```python
from build123d import *

# Parameters (mm, degrees)
REVOLVE1_ANGLE          = 180
SKETCH2_R               = 2.25
CUT_EXTRUDE1_DEPTH      = 15
CUT_EXTRUDE2_DEPTH      = 5
CUT_EXTRUDE2_DEPTH_BACK = 32.176914536
SKETCH4_W               = 3
SKETCH4_H               = 7


with BuildPart() as part:
    # Sketch1 → Revolve1 (revolve)
    with BuildSketch(Plane(origin=(0, 0, 0), x_dir=(0, 0, -1), z_dir=(1, 0, 0))):
        with BuildLine():
            Line((-18, 0), (18, 0))
            ThreePointArc((18, 0), (0, -18), (-18, 0))
        make_face()
    revolve(axis=Axis((0, 0, 18), (0, 0, -1)), revolution_arc=REVOLVE1_ANGLE)

    # Sketch2 → Cut-Extrude1 (cut)
    with BuildSketch(Plane(origin=(0, 0, 0), x_dir=(0, 0, -1), z_dir=(1, 0, 0))):
        with Locations(Location((0, 0, 0), (0, 0, 90))):
            Circle(SKETCH2_R)
    extrude(amount=-CUT_EXTRUDE1_DEPTH, mode=Mode.SUBTRACT)

    # Sketch4 → Cut-Extrude2 (cut, two sides: drawn at the far end of the back side and taken through both)
    with BuildSketch(Plane(origin=(0, 0, 0), x_dir=(1, 0, 0), z_dir=(0, 1, 0)).offset(-CUT_EXTRUDE2_DEPTH_BACK)):
        with Locations((-7.141823204, 0)):
            Rectangle(SKETCH4_W, SKETCH4_H)
    extrude(amount=CUT_EXTRUDE2_DEPTH + CUT_EXTRUDE2_DEPTH_BACK, mode=Mode.SUBTRACT)


solid = part.part
```
Read the model definition and answer for the solid it produces. Units are mm, in the model's axes. A direction names the side the tool comes from. Round coordinates to 2 decimals unless told otherwise and drop trailing zeros. Write each loop counter-clockwise with the first axis right and the second up, starting at its lowest first coordinate (ties: lowest second). Pieces come first, ordered by that corner, then holes. Notation, with made-up numbers: (-16.5, 27) - (6.5, 27) arc R27 ccw to (6.5, 57) - close; hole circle Ø11 at (78, 86.25). An arc over 180 degrees is marked (long way). Use CSV: the item, a comma, the result in double quotes.
Q1. Find section C-C, the plane y = -13.5. Write down the section's boundary in (x, z), then the cut area to 3 significant figures.
Values:
outline,"(0, -11.91) - (0, 11.91) arc R11.91 ccw to start; hole (-8.64, -3.5) - (-5.64, -3.5) - (-5.64, 3.5) - (-8.64, 3.5) - close"
area,"202 mm²"
Q2. Straight lines are drawn through the part: line 1 along Z through (x, y) = (-7, -15); line 2 along Z through (x, y) = (-11.75, 0); line 3 along X through (y, z) = (-8, 0.5). For each, find the intervals that lie inside material, in ascending order.
Values:
line 1,"z = -7.07 to -3.5, 3.5 to 7.07"
line 2,"z = -13.64 to -2.25, 2.25 to 13.64"
line 3,"x = -16.12 to -8.64, -5.64 to 0"
Q3. Each of these flat-tipped pins is pushed along its axis until it touches: pin 1 Ø1.5 at (x, z) = (-14, 0.5) entering from -Y; pin 2 Ø2.5 at (y, z) = (0, 0) entering from +X; pin 3 Ø2 at (y, z) = (-6.5, -0.5) entering from -X; pin 4 Ø1.5 at (x, z) = (-15.5, 13.5) entering from -Y. Where does it stop, or does it pass through?
Values:
pin 1,"stops at y = -12.17"
pin 2,"stops at x = -15"
pin 3,"stops at x = -17.13"
pin 4,"passes through"
Q4. Determine the mould class of faces 3 (the cylindrical face through (-2.781, 2.146, 0.676)), 4 (the flat face through (0, -4, 0)) for opening direction Z: +Z half, -Z half, draft (parallel to the pull), parting line (faces both ways), or undercut.
Values:
face 3,"undercut"
face 4,"draft"
Q5. Find section D-D, the plane x = -5. Write down the section's boundary in (y, z), then the cut area to 3 significant figures.
Values:
outline,"circle Ø34.58 at (0, 0); hole circle Ø4.5 at (0, 0)"
area,"923 mm²"
Q6. Find section A-A, the plane z = 0. Write down the section's boundary in (x, y).
Values:
outline,"(-15, -2.25) - (-15, 2.25) - (-8.64, 2.25) - (-8.64, 5) - (-5.64, 5) - (-5.64, 2.25) - (0, 2.25) - (0, 18) arc R18 ccw to (-8.64, -15.79) - (-8.64, -2.25) - close; (-5.64, -17.09) arc R18 ccw to (0, -18) - (0, -2.25) - (-5.64, -2.25) - close"
Q7. Find section B-B, the plane y = 0. Write down the section's boundary in (x, z), then the cut area to 3 significant figures.
Values:
outline,"(-15, -2.25) - (-15, 2.25) - (-8.64, 2.25) - (-8.64, 3.5) - (-5.64, 3.5) - (-5.64, 2.25) - (0, 2.25) - (0, 18) arc R18 ccw to (0, -18) - (0, -2.25) - (-5.64, -2.25) - (-5.64, -3.5) - (-8.64, -3.5) - (-8.64, -2.25) - close"
area,"434 mm²"
Q8. A tool of negligible diameter and unlimited length cuts with its end or side. For faces 1 (the flat face through (-15, 0, 0)), 2 (the flat face through (-8.642, -6, 0)), from which of +Z, -Z, +X, -X, +Y, -Y can it reach the whole face along a straight path? Write none if from no direction.
Values:
face 1,"+X"
face 2,"-Y"
